Read the model definition and answer for the solid it produces. Units are mm, in the model's axes. A direction names the side the tool comes from. Give positions to 0.01 mm unless a question says otherwise; leave off trailing zeros. Write each loop counter-clockwise with the first axis right and the second up, starting at its lowest first coordinate (ties: lowest second). Pieces come first, ordered by that corner, then holes. Notation, with made-up numbers: M 1,64 L 19,64 A34 ccw 19,95 Z; hole C 22,22.5 d10. An arc over 180 degrees is marked long. Answer as CSV lines item,"result". Start each with the question number.
```python
from build123d import *

# Parameters (mm, degrees)
SKETCH_1_R          = 2.5
SKETCH_1_R_2        = 2
EXTRUDE_1_DEPTH     = 4
SKETCH_2_R          = 2
CUT_EXTRUDE_1_DEPTH = 10
SKETCH_4_R          = 4
CUT_EXTRUDE_2_DEPTH = 3


with BuildPart() as part:
    # 草图1 → 凸台-拉伸1 (new body)
    with BuildSketch(Plane.XY):
        with BuildLine():
            Line((-75.538677918, 13.9), (52.461322082, 13.9))
            Line((52.461322082, 13.9), (65.422072845, 13.9))
            Line((65.422072845, 13.9), (67.422072845, 13.9))
            ThreePointArc((67.422072845, 13.9), (68.129179626, 13.607106781), (68.422072845, 12.9))
            Line((68.422072845, 12.9), (68.422072845, 10.9))
            Line((68.422072845, 10.9), (68.422072845, -12.95))
            ThreePointArc((68.422072845, -12.95), (68.129179626, -13.657106781), (67.422072845, -13.95))
            Line((67.422072845, -13.95), (52.461322082, -13.95))
            Line((52.461322082, -13.95), (52.461322082, -13.9))
            Line((52.461322082, -13.9), (-75.538677918, -13.9))
            Line((-75.538677918, -13.9), (-92.538677918, -13.9))
            Line((-92.538677918, -13.9), (-92.538677918, 13.9))
            Line((-92.538677918, 13.9), (-75.538677918, 13.9))
        make_face()
        with Locations((-75.538677918, 0)):
            Circle(SKETCH_1_R, mode=Mode.SUBTRACT)
        with Locations((52.461322082, 0)):
            Circle(SKETCH_1_R_2, mode=Mode.SUBTRACT)
        with Locations((-43.538677918, 0)):
            Circle(SKETCH_1_R, mode=Mode.SUBTRACT)
    extrude(amount=EXTRUDE_1_DEPTH)

    # 草图2 → 切除-拉伸1 (cut)
    with BuildSketch(Plane(origin=(0, 0, 0), x_dir=(-1, 0, 0), z_dir=(0, 0, -1))):
        with Locations((-52.461322082, -9)):
            Circle(SKETCH_2_R)
        with Locations((-52.461322082, 9)):
            Circle(SKETCH_2_R)
    extrude(amount=-CUT_EXTRUDE_1_DEPTH, mode=Mode.SUBTRACT)

    # 草图4 → 切除-拉伸2 (cut)
    with BuildSketch(Plane.XY.offset(4)):
        with Locations((-43.538677918, 0)):
            Circle(SKETCH_4_R)
    extrude(amount=-CUT_EXTRUDE_2_DEPTH, mode=Mode.SUBTRACT)


solid = part.part
```
1. Determine the mould class of faces 1 (the face through (-92.539, 0, 2)), 2 (the face through (68.422, 0, 2)), 3 (the face through (-41.23, -0.96, 0.49)), 4 (the face through (-73.154, 0.751, 1.972)) for opening direction X: +X half, -X half, draft (parallel to the pull), parting line (faces both ways), or undercut.
2. For faces 5 (the face through (-44, -3, 1)), 6 (the face through (60, -13.95, 2)), determine the directions among +Z, -Z, +X, -X, +Y, -Y from which every point of the face is accessible in a straight line to the end or side of a thin tool.
3. Find section A-A on y = -9. Determine the outline of the cut face in (x, z).
4. Find the intervals of material crossed by line 1 (X direction, y = -0.25, z = 2.55); line 2 (X direction, y = -9.25, z = 2.05); line 3 (Y direction, x = -57.5, z = 3.65), in increasing order. Write a range as [from, to].
5. Given pin 1 (2 mm diameter, centred on x = -44, z = 2, fed in from -Y), flat-ended and moving along its own axis, determine where the tip first touches the part or whether it passes through.
6. Find section C-C on y = 0. Determine the outline of the cut face in (x, z), then the cut area to 3 significant figures.
7. Find section B-B on z = 2.3. Determine the outline of the cut face in (x, y).
Computed:
1,face 1,"-X half"
1,face 2,"+X half"
1,face 3,"undercut"
1,face 4,"undercut"
2,face 5,"+Z"
2,face 6,"+Z, -Z, +X, -X, -Y"
3,outline,"M -92.54,0 L 50.46,0 L 50.46,4 L -92.54,4 Z; M 54.46,0 L 68.42,0 L 68.42,4 L 54.46,4 Z"
4,line 1,"x = [-92.54, -78.03], [-73.05, -47.53], [-39.55, 50.48], [54.45, 68.42]"
4,line 2,"x = [-92.54, 50.48], [54.45, 68.42]"
4,line 3,"y = [-13.9, 13.9]"
5,pin 1,"stops at y = -13.9"
6,outline,"M -92.54,0 L -78.04,0 L -78.04,4 L -92.54,4 Z; M -73.04,0 L -46.04,0 L -46.04,1 L -47.54,1 L -47.54,4 L -73.04,4 Z; M -41.04,0 L 50.46,0 L 50.46,4 L -39.54,4 L -39.54,1 L -41.04,1 Z; M 54.46,0 L 68.42,0 L 68.42,4 L 54.46,4 Z"
6,area,"579 mm^2"
7,outline,"M -92.54,-13.9 L 52.46,-13.9 L 52.46,-13.95 L 67.42,-13.95 A1 ccw 68.42,-12.95 L 68.42,12.9 A1 ccw 67.42,13.9 L -92.54,13.9 Z; hole C -75.54,0 d5; hole C -43.54,0 d8; hole C 52.46,-9 d4; hole C 52.46,0 d4; hole C 52.46,9 d4"
